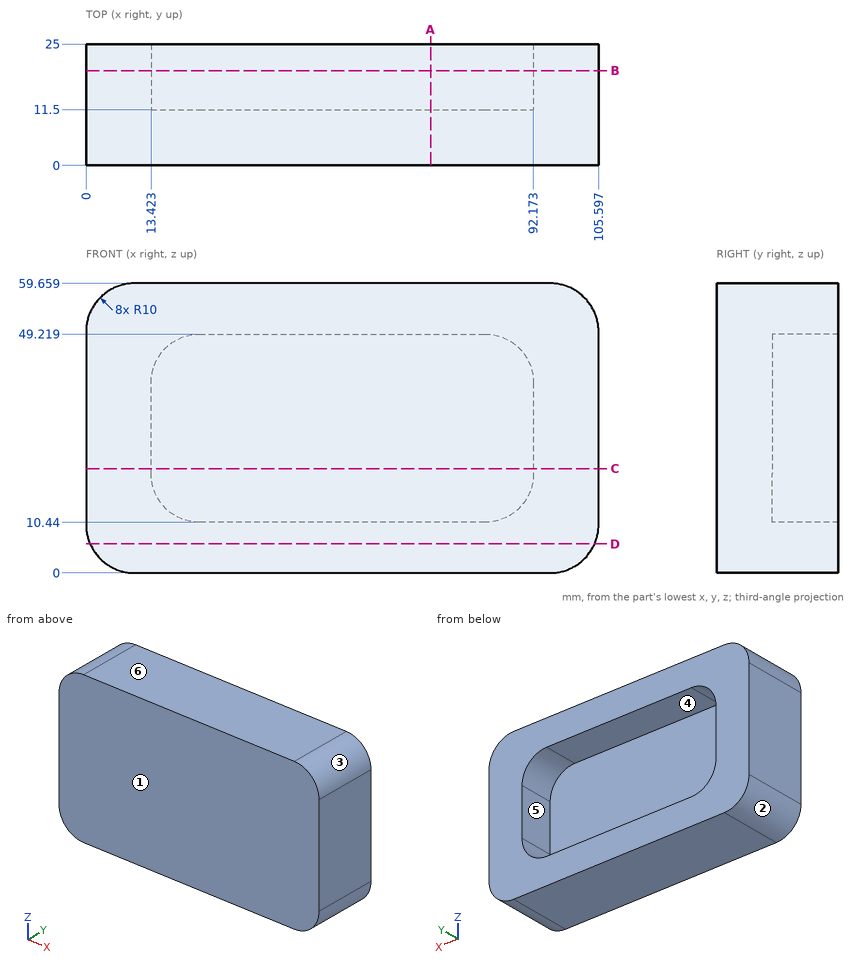
For this review, use the dimensioned drawing (mm, ordinates from the lowest corner) and the shaded views. A direction names the side the tool comes from. Round coordinates to 2 decimals unless told otherwise and drop trailing zeros. Write each loop counter-clockwise with the first axis right and the second up, starting at its lowest first coordinate (ties: lowest second). Pieces come first, ordered by that corner, then holes. Notation, with made-up numbers: (71.5, 10) - (77.5, 10) arc R23 cw to (77.5, 41) - close; hole circle Ø6 at (1, -11). An arc over 180 degrees is marked (long way). Answer as a JSON object with one key per item and string values.
1. We need section C-C on z = 21.5. Give the boundary of the cut face in (x, y), then the cut area to 3 significant figures.
Response values:
{"outline": "(0, 0) - (105.6, 0) - (105.6, 25) - (92.17, 25) - (92.17, 11.5) - (13.42, 11.5) - (13.42, 25) - (0, 25) - close", "area": "1,580 mm2"}
2. We need section A-A on x = 71. Give the boundary of the cut face in (y, z).
Response values:
{"outline": "(0, 0) - (25, 0) - (25, 10.44) - (11.5, 10.44) - (11.5, 49.22) - (25, 49.22) - (25, 59.66) - (0, 59.66) - close"}
3. Tool access review of the marked faces 5 and 6: name each direction out of +Z, -Z, +X, -X, +Y, -Y from which nothing blocks a thin tool from reaching the whole face with its end or side.
Response values:
{"face 5": "+Y", "face 6": "+Z, +X, -X, +Y, -Y"}
4. We need section D-D on z = 6. Give the boundary of the cut face in (x, y) (1 decimal), then the cut area to 3 significant figures.
Response values:
{"outline": "(0.8, 0) - (104.8, 0) - (104.8, 25) - (0.8, 25) - close", "area": "2,600 mm2"}
5. For pin 1 Ø19.5 at (x, z) = (42.5, 24) entering from +Y, flat-tipped, find the tip position at first contact; note if it passes through.
Response values:
{"pin 1": "stops at y = 11.5"}
6. We need section B-B on y = 19.5. Give the boundary of the cut face in (x, z).
Response values:
{"outline": "(0, 10) arc R10 ccw to (10, 0) - (95.6, 0) arc R10 ccw to (105.6, 10) - (105.6, 49.66) arc R10 ccw to (95.6, 59.66) - (10, 59.66) arc R10 ccw to (0, 49.66) - close; hole (13.42, 20.44) arc R10 ccw to (23.42, 10.44) - (82.17, 10.44) arc R10 ccw to (92.17, 20.44) - (92.17, 39.22) arc R10 ccw to (82.17, 49.22) - (23.42, 49.22) arc R10 ccw to (13.42, 39.22) - close"}
7. Draft analysis for pull direction X (two halves, no side actions). For the marked faces 1, 2, 3 and 4, state which applies: +X half, -X half, draft (parallel to the pull), parting line (faces both ways), or undercut.
Response values:
{"face 1": "draft", "face 2": "-X half", "face 3": "+X half", "face 4": "undercut"}
8. To check wall thickness, follow line 1 along Z through (x, y) = (34, 20.25); line 2 along X through (y, z) = (13.5, 37.5); line 3 along Y through (x, z) = (19.5, 14). State the ranges of each line that lie inside material, in increasing order.
Response values:
{"line 1": "z = 0 to 10.44, 49.22 to 59.66", "line 2": "x = 0 to 13.42, 92.17 to 105.6", "line 3": "y = 0 to 11.5"}
